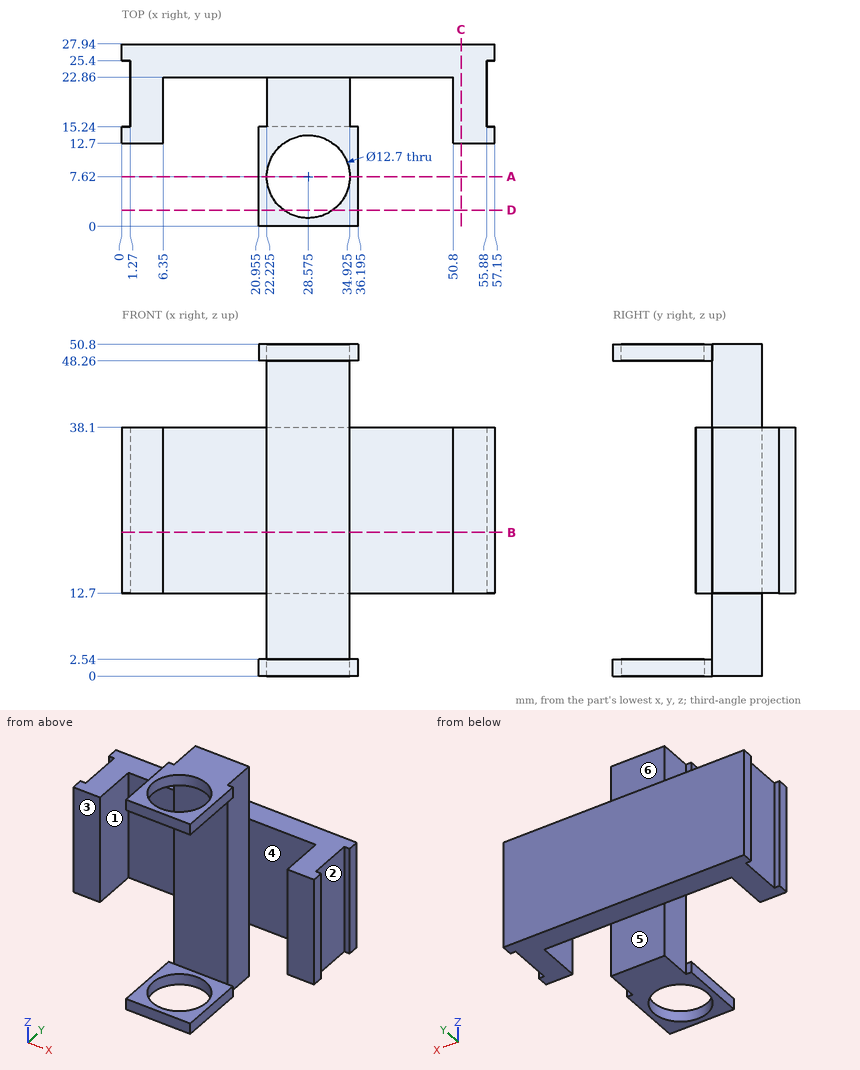
Geometry: see drawing. Coordinates: mm, zero at the bounding-box minimum. A direction names the side the tool comes from. Give positions to 0.01 mm unless a question says otherwise; leave off trailing zeros. Write each loop counter-clockwise with the first axis right and the second up, starting at its lowest first coordinate (ties: lowest second). Pieces come first, ordered by that corner, then holes. Notation, with made-up numbers: (-36.75, 84) - (21.25, 84) arc R23 ccw to (21.25, 94) - close; hole circle Ø1 at (-1.5, 30.5). An arc over 180 degrees is marked (long way). Return JSON: item names as keys, results as strings. Group by question number.
1) First-contact query: P1, Ø5, axis at y = 11, z = 9.5, coming from the -X side; P2, Ø1, axis at y = 23, z = 24.5, coming from the +X side; P3, Ø5, axis at x = 44.5, z = 20.5, coming from the -Y side; P4, Ø2, axis at y = 7, z = 50, coming from the -X side (3 decimals). Flat tips, straight axial feed; report the tip coordinate or a pass-through.
2) Section A-A on y = 7.62. Return the cut outline in (x, z) (3 decimals).
3) Line query: line 1 (X direction, y = 19.5, z = 22) (3 decimals); line 2 (Z direction, x = 25, y = 14.5); line 3 (Y direction, x = 30, z = 9.5). Output: solid intervals per line, ascending.
4) Section B-B on z = 22. Return the cut outline in (x, y) (3 decimals).
5) Section C-C on x = 52. Return the cut outline in (y, z).
6) Set-up query: the marked faces 4, 5 and 6. Return all of +Z, -Z, +X, -X, +Y, -Y with unobstructed straight access to the full face (end or side cutting, diameter ignored); none if empty.
7) Mould query, pull axis X, two halves, no side actions, for the marked faces 1, 2 and 3. Classes: released by +X, released by -X, zero draft, split by the parting line, or undercut.
8) Section D-D on y = 2.5. Return the cut outline in (x, z) (3 decimals), plus the area to 3 significant figures.
Filled in:
{
 "1": {"P1": "passes through", "P2": "stops at x = 55.88", "P3": "stops at y = 22.86", "P4": "stops at x = 20.955"},
 "2": {"outline": "(20.955, 0) - (22.225, 0) - (22.225, 2.54) - (20.955, 2.54) - close; (20.955, 48.26) - (22.225, 48.26) - (22.225, 50.8) - (20.955, 50.8) - close; (34.925, 0) - (36.195, 0) - (36.195, 2.54) - (34.925, 2.54) - close; (34.925, 48.26) - (36.195, 48.26) - (36.195, 50.8) - (34.925, 50.8) - close"},
 "3": {"line 1": "x = 1.27 to 6.35, 22.225 to 34.925, 50.8 to 55.88", "line 2": "z = 0 to 2.54, 48.26 to 50.8", "line 3": "y = 15.24 to 22.86"},
 "4": {"outline": "(0, 12.7) - (6.35, 12.7) - (6.35, 22.86) - (22.225, 22.86) - (22.225, 15.24) - (34.925, 15.24) - (34.925, 22.86) - (50.8, 22.86) - (50.8, 12.7) - (57.15, 12.7) - (57.15, 15.24) - (55.88, 15.24) - (55.88, 25.4) - (57.15, 25.4) - (57.15, 27.94) - (0, 27.94) - (0, 25.4) - (1.27, 25.4) - (1.27, 15.24) - (0, 15.24) - close"},
 "5": {"outline": "(12.7, 12.7) - (27.94, 12.7) - (27.94, 38.1) - (12.7, 38.1) - close"},
 "6": {"face 4": "+Z, -Z, -Y", "face 5": "-Z, +X, -X, +Y", "face 6": "+Z, +X, -X, +Y"},
 "7": {"face 1": "undercut", "face 2": "released by +X", "face 3": "zero draft"},
 "8": {"outline": "(20.955, 0) - (24.819, 0) - (24.819, 2.54) - (20.955, 2.54) - close; (20.955, 48.26) - (24.819, 48.26) - (24.819, 50.8) - (20.955, 50.8) - close; (32.331, 0) - (36.195, 0) - (36.195, 2.54) - (32.331, 2.54) - close; (32.331, 48.26) - (36.195, 48.26) - (36.195, 50.8) - (32.331, 50.8) - close", "area": "39.3 mm^2"}
}
